from build123d import *

# Parameters (mm, degrees)
F0_R      = 7.9375
F1_DEPTH  = 25.4
F2_R      = 4.7625
F3_DEPTH  = 6.35
F4_W      = 7
F4_H      = 7
F5_DEPTH  = 25.4
F6_W      = 3
F6_H      = 3
F7_DEPTH  = 25.4
F9_W      = 15.748512
F9_H      = 2
F10_DEPTH = 25.4
F12_W     = 2.079316
F12_H     = 12.7
F13_DEPTH = 25.4
F15_R     = 7.9375
F15_R_2   = 3.5
F16_DEPTH = 2


with BuildPart() as f1:
    # F0 (on Top) → F1 (new body)
    with BuildSketch(Plane.XY):
        Circle(F0_R)
    extrude(amount=F1_DEPTH)

    # F2 (on Top) → F3 (join)
    with BuildSketch(Plane.XY):
        Circle(F2_R)
    extrude(amount=-F3_DEPTH)

    # F4 (on face) → F5 (join)
    with BuildSketch(Plane.XY.offset(25.4)):
        Rectangle(F4_W, F4_H)
    extrude(amount=F5_DEPTH)


with BuildPart() as f7:
    # F6 (on face) → F7 (new body)
    with BuildSketch(Plane.XY.offset(25.4)):
        Rectangle(F6_W, F6_H)
    extrude(amount=F7_DEPTH)


with BuildPart() as f1_1:
    add(f1.part)

    # F8: cut F7
    add(f7.part, mode=Mode.SUBTRACT)


with BuildPart() as f10:
    # F9 (on face) → F10 (new body)
    with BuildSketch(Plane.XY.offset(25.4)):
        Rectangle(F9_W, F9_H)
    extrude(amount=F10_DEPTH)


with BuildPart() as f1_2:
    add(f1_1.part)

    # F11: cut F10
    add(f10.part, mode=Mode.SUBTRACT)


with BuildPart() as f13:
    # F12 (on face) → F13 (new body)
    with BuildSketch(Plane.XZ.offset(3.5)):
        with Locations((0, 19.05)):
            Rectangle(F12_W, F12_H)
    extrude(amount=F13_DEPTH)


with BuildPart() as f1_3:
    add(f1_2.part)

    # F14: cut F13
    add(f13.part, mode=Mode.SUBTRACT)


with BuildPart() as f16:
    # F15 (on face) → F16 (new body)
    with BuildSketch(Plane.XY.offset(12.7)):
        Circle(F15_R)
        Circle(F15_R_2, mode=Mode.SUBTRACT)
    extrude(amount=F16_DEPTH)


with BuildPart() as f1_4:
    add(f1_3.part)

    # F17: cut F16
    add(f16.part, mode=Mode.SUBTRACT)


solid = f1_4.part
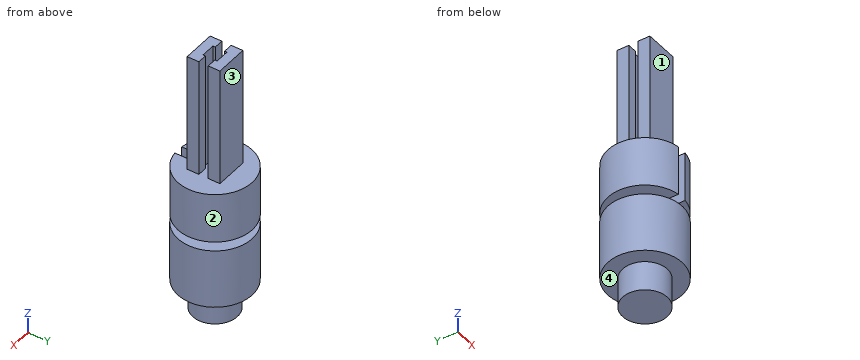
Geometry: final body of the model. Coordinates: model frame, mm. Face numbers are marked on the shaded views. A direction names the side the tool comes from. Round coordinates to 2 decimals unless told otherwise and drop trailing zeros. Loops run counter-clockwise (first coordinate to the right, second up) from the corner with the lowest first, then second, coordinate; pieces in that order, holes last. Notation, with made-up numbers: (-29, 87) - (23, 87) arc R35 cw to (23, 122) - close; hole circle Ø2 at (67, 47). An arc over 180 degrees is marked (long way). Write each question's results on one line, items separated by ' | '. Start each with the question number.
1) First-contact query: P1, Ø3.5, axis at y = -5.5, z = 17.5, coming from the -X side; P2, Ø1.5, axis at x = 6, z = 34, coming from the +Y side; P3, Ø1.2, axis at y = 2.5, z = 36.5, coming from the +X side; P4, Ø8, axis at x = 1, z = 32, coming from the -Y side. Flat tips, straight axial feed; report the tip coordinate or a pass-through.
2) Cut plane D-D on x = -2. Return loops of the section in (y, z), then the cut area to 3 significant figures.
3) Cut plane B-B on y = 0. Return loops of the section in (x, z), then the cut area to 3 significant figures.
4) Line query: probe 1 along Y at (x, z) = (-2.5, 45.5); probe 2 along Z at (x, y) = (-5, -3.5); probe 3 along Z at (x, y) = (4.5, -0.5). Output: solid intervals per line, ascending. Write a range as [from, to].
5) Cut plane C-C on x = 6. Return loops of the section in (y, z).
6) Access query for the marked faces 1, 2, 3 and 4. Directions: +Z, -Z, +X, -X, +Y, -Y. A direction counts if a zero-diameter tool reaches every point of the face in a straight line with its end or side. Return the directions, or none.
7) Cut plane A-A on z = 44.5. Return loops of the section in (x, y), then the cut area to 3 significant figures.
Verdict:
1) P1: stops at x = -7 | P2: passes through | P3: stops at x = 3.5 | P4: stops at y = -3.5
2) outline: (-7.68, 0) - (-4.32, 0) - (-4.32, -6.35) - (4.32, -6.35) - (4.32, 0) - (7.68, 0) - (7.68, 12.7) - (2.87, 12.7) - (2.87, 14.7) - (7.68, 14.7) - (7.68, 25.4) - (3.5, 25.4) - (3.5, 50.8) - (1, 50.8) - (1, 25.4) - (-1, 25.4) - (-1, 50.8) - (-3.5, 50.8) - (-3.5, 25.4) - (-7.68, 25.4) - (-7.68, 14.7) - (-2.87, 14.7) - (-2.87, 12.7) - (-7.68, 12.7) - close | area: 553 mm2
3) outline: (-7.94, 0) - (-4.76, 0) - (-4.76, -6.35) - (4.76, -6.35) - (4.76, 0) - (7.94, 0) - (7.94, 12.7) - (3.5, 12.7) - (3.5, 14.7) - (7.94, 14.7) - (7.94, 25.4) - (-7.94, 25.4) - (-7.94, 14.7) - (-3.5, 14.7) - (-3.5, 12.7) - (-7.94, 12.7) - close | area: 446 mm2
4) probe 1: y = [-3.5, -1], [1, 3.5] | probe 2: z = [0, 12.7], [14.7, 25.4] | probe 3: z = [-6.35, 12.7], [14.7, 25.4]
5) outline: (-5.2, 0) - (5.2, 0) - (5.2, 12.7) - (-5.2, 12.7) - close; (-5.2, 14.7) - (5.2, 14.7) - (5.2, 25.4) - (-5.2, 25.4) - close
6) face 1: +Z, -Y | face 2: +Z, -Z | face 3: +Z, +X, -X, +Y | face 4: -Z
7) outline: (-3.5, -3.5) - (3.5, -3.5) - (3.5, -1) - (1.5, -1) - (1.5, -1.5) - (-1.5, -1.5) - (-1.5, -1) - (-3.5, -1) - close; (-3.5, 1) - (-1.5, 1) - (-1.5, 1.5) - (1.5, 1.5) - (1.5, 1) - (3.5, 1) - (3.5, 3.5) - (-3.5, 3.5) - close | area: 32.0 mm2
